Source: CAD feature listing. Evaluate the final solid. Frame: model axes, mm. A direction names the side the tool comes from. Round coordinates to 2 decimals unless told otherwise and drop trailing zeros. Write each loop counter-clockwise with the first axis right and the second up, starting at its lowest first coordinate (ties: lowest second). Pieces come first, ordered by that corner, then holes.
from build123d import *

# Parameters (mm, degrees)
BOSS_EXTRUDE1_DEPTH = 40
SKETCH3_W           = 185.690324397
SKETCH3_H           = 500
BOSS_EXTRUDE2_DEPTH = 30
SKETCH4_R           = 34.175984335
CUT_EXTRUDE1_DEPTH  = 30
LPATTERN1_COUNT     = 2
LPATTERN1_PITCH     = 200
LPATTERN1_COL_COUNT = 2
LPATTERN1_COL_PITCH = 200


with BuildPart() as part:
    # Sketch1 → Boss-Extrude1 (new body)
    with BuildSketch(Plane(origin=(0, 0, 0), x_dir=(1, 0, 0), z_dir=(0, 1, 0))):
        Polygon((-46.422581099, 32.577249894), (-147.004840148, -54.974109197), (46.422581099, -32.577249894), (46.422581099, 32.577249894), align=None)
    boss_extrude1 = extrude(amount=BOSS_EXTRUDE1_DEPTH)

    # Mirror1: Boss-Extrude1 across plane
    add(boss_extrude1.mirror(Plane(origin=(46.422581099, 40, -32.577249894), x_dir=(0, 0, 1), z_dir=(-1, 0, 0))))

    # Sketch3 → Boss-Extrude2 (add)
    with BuildSketch(Plane(origin=(0, 0, -32.577249894), x_dir=(-1, 0, 0), z_dir=(0, 0, -1))):
        with Locations((-46.422581099, 250)):
            Rectangle(SKETCH3_W, SKETCH3_H)
    extrude(amount=BOSS_EXTRUDE2_DEPTH)

    # Mirror5: Boss-Extrude1 across plane
    add(boss_extrude1.mirror(Plane.ZX.offset(250)))

    # Sketch4 → Cut-Extrude1 (cut)
    with BuildSketch(Plane(origin=(0, 0, -62.577249894), x_dir=(-1, 0, 0), z_dir=(0, 0, -1))):
        with Locations((-46.422581099, 250)):
            Circle(SKETCH4_R)
    cut_extrude1 = extrude(amount=-CUT_EXTRUDE1_DEPTH, mode=Mode.SUBTRACT)

    # LPattern1: Cut-Extrude1 ×2
    with Locations(*[(0, i * LPATTERN1_PITCH, 0) for i in range(1, LPATTERN1_COUNT)]):
        add(cut_extrude1, mode=Mode.SUBTRACT)

    # LPattern1 col: Cut-Extrude1 ×2
    with Locations(*[(0, -i * LPATTERN1_COL_PITCH, 0) for i in range(1, LPATTERN1_COL_COUNT)]):
        add(cut_extrude1, mode=Mode.SUBTRACT)


solid = part.part
1) Contact query for flat-ended pins moving along their axis: P1, Ø20, axis at y = 486.5, z = -12.5, coming from the +X side; P2, Ø2, axis at y = 134, z = -48.5, coming from the +X side; P3, Ø15, axis at y = 241.5, z = -44, coming from the -X side. Output: stop coordinate, or through.
Taken from the geometry:
P1: stops at x = 46.42
P2: stops at x = 139.27
P3: stops at x = -46.42
2) Reachability of faces 1 (the face through (-46.423, 247, -47)), 2 (the face through (49, 40, 11)), 3 (the face through (13.825, 60.266, -47.787)), 4 (the face through (-51.645, 19.72, 43.932)) from +Z, -Z, +X, -X, +Y, -Y: full face, straight path, thin tool, end or side. Return the list, or none.
Taken from the geometry:
face 1: -Z, -X, +Y, -Y
face 2: +Z, +X, -X
face 3: -Z
face 4: +Z, +Y, -Y
3) Material intervals for line 1 (Y direction, x = 35, z = 22); line 2 (X direction, y = 450, z = -41); line 3 (Y direction, x = 38, z = -37), sorted ascending.
Taken from the geometry:
line 1: y = 0 to 40, 460 to 500
line 2: x = -46.42 to 12.25, 80.6 to 139.27
line 3: y = 0 to 16.88, 83.12 to 216.88, 283.12 to 416.88, 483.12 to 500
4) Section query B-B on y = 450. Return the cut outline in (x, z).
Taken from the geometry:
outline: (-46.42, -62.58) - (12.25, -62.58) - (12.25, -32.58) - (-46.42, -32.58) - close; (80.6, -62.58) - (139.27, -62.58) - (139.27, -32.58) - (80.6, -32.58) - close
5) Pull-direction query (X, two-part tool) for faces 5 (the face through (188.855, 19.72, 10.586)), 6 (the face through (34, 470, -32.577)), 7 (the face through (-96.01, 19.72, 10.586)); classes: released by +X, released by -X, zero draft, split by the parting line, or undercut.
Taken from the geometry:
face 5: released by +X
face 6: undercut
face 7: released by -X
6) Section query C-C on y = 157. Return the cut outline in (x, z).
Taken from the geometry:
outline: (-46.42, -62.58) - (139.27, -62.58) - (139.27, -32.58) - (-46.42, -32.58) - close
7) Section query A-A on z = -23.5. Return the cut outline in (x, y), then the cut area to 3 significant figures.
Taken from the geometry:
outline: (-56.85, 0) - (149.7, 0) - (149.7, 40) - (-56.85, 40) - close; (-56.85, 460) - (46.42, 460) - (46.42, 500) - (-56.85, 500) - close
area: 12,400 mm2
